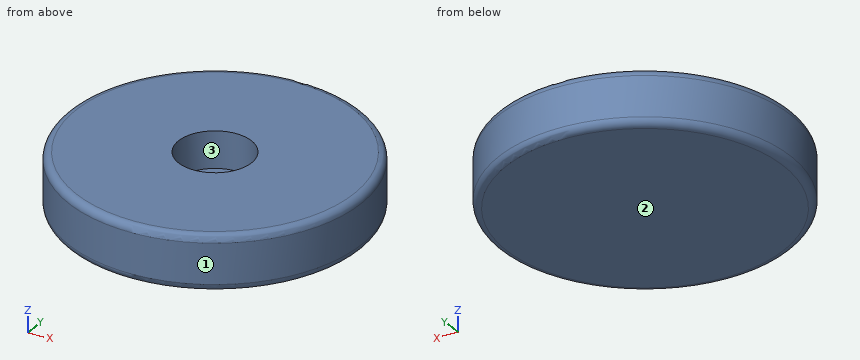
from build123d import *

# Parameters (mm, degrees)
SKETCH1_R          = 101.6
WHEEL_DEPTH        = 19.05
FILLET1_R          = 5.08
SKETCH2_R          = 25.4
CUT_EXTRUDE1_DEPTH = 25.4


with BuildPart() as part:
    # Sketch1 → Wheel (new body, symmetric)
    with BuildSketch(Plane.XY):
        Circle(SKETCH1_R)
    extrude(amount=WHEEL_DEPTH, both=True)

    # Fillet1
    fillet1_edges = [part.edges().sort_by_distance(p)[0] for p in [
        (-101.6, 0, -19.05),
        (-101.6, 0, 19.05),
    ]]
    fillet(fillet1_edges, radius=FILLET1_R)

    # Sketch2 → Cut-Extrude1 (cut)
    with BuildSketch(Plane.XY.offset(19.05)):
        Circle(SKETCH2_R)
    extrude(amount=-CUT_EXTRUDE1_DEPTH, mode=Mode.SUBTRACT)


solid = part.part
Source: CAD feature listing. Evaluate the final solid. Frame: model axes, mm. Face numbers are marked on the shaded views. Coordinates: 2 decimals unless noted, no trailing zeros. Loops run counter-clockwise (first coordinate to the right, second up) from the corner with the lowest first, then second, coordinate; pieces in that order, holes last. Notation, with made-up numbers: (37.5, 36.5) - (88.5, 36.5) arc R14 cw to (88.5, 44.5) - close; hole circle Ø6 at (-17.5, 19.5). An arc over 180 degrees is marked (long way). Return JSON: item names as keys, results as strings.
Q1. Section C-C, the plane z = 5. Return loops of the section in (x, y), plus the area to 3 significant figures.
Results:
{"outline": "circle Ø203.2 at (0, 0); hole circle Ø50.8 at (0, 0)", "area": "30,400 mm2"}
Q2. Mould query, pull axis X, two halves, no side actions, for the marked faces 1, 2 and 3. Classes: released by +X, released by -X, zero draft, split by the parting line, or undercut.
Results:
{"face 1": "split by the parting line", "face 2": "zero draft", "face 3": "undercut"}
Q3. Section A-A, the plane x = 0. Return loops of the section in (y, z).
Results:
{"outline": "(-101.6, -13.97) arc R5.08 ccw to (-96.52, -19.05) - (96.52, -19.05) arc R5.08 ccw to (101.6, -13.97) - (101.6, 13.97) arc R5.08 ccw to (96.52, 19.05) - (25.4, 19.05) - (25.4, -6.35) - (-25.4, -6.35) - (-25.4, 19.05) - (-96.52, 19.05) arc R5.08 ccw to (-101.6, 13.97) - close"}
Q4. Contact query for flat-ended pins moving along their axis: P1, Ø3, axis at y = -40.5, z = 0, coming from the +X side; P2, Ø3, axis at y = -75, z = -2.5, coming from the +X side; P3, Ø1.5, axis at x = 40.5, z = 1.5, coming from the +Y side. Output: stop coordinate, or through.
Results:
{"P1": "x = 93.82", "P2": "x = 70.14", "P3": "y = 93.5"}
Q5. Material intervals for line 1 along Y through (x, z) = (0, 7); line 2 along X through (y, z) = (-17, 5); line 3 along Y through (x, z) = (14, 11), sorted ascending.
Results:
{"line 1": "-101.6 to -25.4, 25.4 to 101.6", "line 2": "-100.17 to -18.87, 18.87 to 100.17", "line 3": "-100.63 to -21.19, 21.19 to 100.63"}
